Autodesk Inventor part; units mm, degrees
ref_plane "YZ Plane" through (0, 0, 0) normal (1, 0, 0) x (0, 1, 0)
ref_plane "XZ Plane" through (0, 0, 0) normal (0, 1, 0) x (-1, 0, 0)
ref_plane "XY Plane" through (0, 0, 0) normal (0, 0, 1) x (1, 0, 0)
sketch "Sketch1" plane through (0, 0, 0) normal (0, 1, 0) x (-1, 0, 0)
  line L0 (12, -6.9282) -> (0, -13.8564)
  line L1 (0, -13.8564) -> (-12, -6.9282)
  line L2 (-12, -6.9282) -> (-12, 6.9282)
  line L3 (-12, 6.9282) -> (0, 13.8564)
  line L4 (0, 13.8564) -> (12, 6.9282)
  line L5 (12, 6.9282) -> (12, -6.9282)
  point P0 (0, 0)
  point P1 (0, 0)
  point P2 (-12, 0)
  point P3 (12, 0)
  dimension "d0" = 24
extrude "Extrusion1" add sketch "Sketch1" along normal blind 10
sketch "Sketch2" plane through (0, 10, 0) normal (0, 1, 0) x (1, 0, 0)
  circle A0 centre (0, 0) radius 12
extrude "Extrusion2" cut sketch "Sketch2" against normal blind 10 draft 60 keep common part
sketch "Sketch3" plane through (0, 0, 0) normal (0, -1, 0) x (1, 0, 0)
  circle A0 centre (0, 0) radius 8
  dimension "d5" = 16
extrude "Extrusion3" add sketch "Sketch3" along normal blind 60
thread "Thread1"
chamfer "Chamfer1" distance 2 angle 45 1 edges at (-8, -60, 0)
fillet "Fillet1" radius 0.6 1 edges at (-8, 0, 0)
properties part number "csavark" material "Steel, Alloy"
For this review, take the finished solid that the model builds, in its own axes (mm). A direction names the side the tool comes from. Round coordinates to 2 decimals unless told otherwise and drop trailing zeros. Write each loop counter-clockwise with the first axis right and the second up, starting at its lowest first coordinate (ties: lowest second). Pieces come first, ordered by that corner, then holes. Notation, with made-up numbers: (37.25, 75.5) - (41.25, 75.5) arc R13 cw to (41.25, 85.5) - close; hole circle Ø6 at (9.25, 0). An arc over 180 degrees is marked (long way). Write item = value, one per line. Start each with the question number.
1. Consider section A-A on y = -19. State the section outline as (x, z) points.
2. For pin 1 Ø12 at (x, y) = (9, -11) entering from +Z; pin 2 Ø6 at (x, y) = (-4.5, -22) entering from -Z; pin 3 Ø4 at (y, z) = (-11.5, -6.5) entering from -X, all flat-tipped, find the tip position at first contact; note any pin that passes through.
3. Draft analysis for pull direction Z (two halves, no side actions). For faces 3 (the face through (5.92, 4.93, -10.44)), 4 (the face through (0.03, 9.74, 12.45)), 5 (the face through (0, 10, 0)), state which applies: released by +Z, released by -Z, zero draft, split by the parting line, or undercut.
4. For faces 1 (the face through (12, 5, 0)), 2 (the face through (-1.73, -28.9, 7.81)), list the 3-axis set-ups (+Z, -Z, +X, -X, +Y, -Y) from which the entire face can be reached by the end or side of a thin tool; tool diameter is ignored.
5. Wall thickness on L1, parallel to Y at x = -9.5, z = -1.75; L2, parallel to Z at x = -0.25, y = -52.5; L3, parallel to Z at x = -4.25, y = -56: over which ranges is each line inside the solid? List them lowest first.
Evaluation:
q1.outline = circle Ø16 at (0, 0)
q2.pin_1 = 7.42
q2.pin_2 = -7.86
q2.pin_3 = -6.61
q3.face_3 = released by -Z
q3.face_4 = released by +Z
q3.face_5 = zero draft
q4.face_1 = +Z, -Z, +X, +Y, -Y
q4.face_2 = -Y
q5.L1 = 0 to 10
q5.L2 = -8 to 8
q5.L3 = -6.78 to 6.78
